Autodesk Inventor part; units mm, degrees
ref_plane "acrylic_sheet_plane" through (0, 0, 4) normal (0, 0, 1) x (1, 0, 0)
ref_plane "YZ Plane" through (0, 0, 0) normal (1, 0, 0) x (0, 1, 0)
ref_plane "XZ Plane" through (0, 0, 0) normal (0, 1, 0) x (-1, 0, 0)
sketch "ferrite_layer_outline_sketch" plane through (0, 0, 0) normal (0, 0, 1) x (1, 0, 0)
  line L0 (-400, 200) -> (400, 200)
  line L1 (400, 200) -> (400, -200)
  line L2 (400, -200) -> (-400, -200)
  line L3 (-400, -200) -> (-400, 200)
  line L4 (0, 200) -> (0, -200) construction
  line L5 (0, 136.1953) -> (0, -273.5408) construction
  line L6 (0, 200) -> (0, -200)
  point P0 (0, 0)
  point P1 (0, 0)
  point P2 (0, 0)
  dimension "d85" = 800
  dimension "d86" = 400
extrude "Sheet Extrude" add sketch "ferrite_layer_outline_sketch" along normal blind 4
ref_plane "acrylic_sheet_plane" through (0, 0, 4) normal (0, 0, 1) x (1, 0, 0)
sketch "Sketch4" plane through (0, 0, 4) normal (0, 0, 1) x (1, 0, 0)
  line L0 (-385.5, 109) -> (-370.5, 109)
  line L1 (-370.5, 109) -> (-370.5, -109)
  line L2 (-370.5, -109) -> (-385.5, -109)
  line L3 (-385.5, -109) -> (-385.5, 109)
  line L4 (-12.6534, 0) -> (47.471, 0)
  line L5 (-400, 200) -> (-400, -200)
  line L6 (400, 200) -> (-400, 200)
  line L7 (-400, -200) -> (400, -200)
  point P0 (0, 0)
  point P1 (-385.5, 0)
  point P2 (-400, 0)
  dimension "d43" = 15
  dimension "d44" = 218
  dimension "d45" = 14.5
extrude "Extrusion9" cut sketch "Sketch4" against normal through all
pattern_linear "Rectangular Pattern 7 fer" count 7 spacing 126 along (1, 0, 0) of "Extrusion9"
pattern_linear "Rectangular Pattern 8 fer" count 8 spacing 108 along (1, 0, 0) of "Extrusion9"
pattern_linear "pattern_test_#_of_ferrites 9 fer" [suppressed]
pattern_linear "Rectangular Pattern 10 fer" [suppressed]
pattern_linear "Rectangular Pattern 13" count 13 spacing 63 along (1, 0, 0) of "Extrusion9"
sketch "dimension_layout_sketch" plane through (0, 0, 4) normal (0, 0, 1) x (1, 0, 0)
  line L0 (-400, 200) -> (-400, -200)
  line L1 (400, -200) -> (400, 200)
  line L2 (400, 200) -> (-400, 200)
  line L3 (-400, -200) -> (400, -200)
  line L4 (-400, 150) -> (400, 150)
  line L5 (400, 150) -> (400, -150)
  line L6 (400, -150) -> (-400, -150)
  line L7 (-400, -150) -> (-400, 150)
  line L8 (0, 150) -> (0, -150) construction
  line L9 (-400, 200) -> (-400, -200) construction
  circle A0 centre (-359.2579, 182.7315) radius 4
  point P0 (0, 0)
  dimension "d87" = 300
  dimension "d88" = 8
sketch "wire_guide_layout_sketch" plane through (0, 0, 4) normal (0, 0, 1) x (1, 0, 0)
  line L0 (-400, -200) -> (400, -200)
  line L1 (-356.5, 92.3814) -> (-350, 92.3814)
  line L2 (-350, 92.3814) -> (-350, -200)
  line L3 (-350, -200) -> (-356.5, -200)
  line L4 (-356.5, -200) -> (-356.5, 92.3814)
  line L5 (-400, 200) -> (-400, -200)
  line L6 (-385.5, 109) -> (-370.5, 109)
  line L7 (-350, -60) -> (-345.5, -60)
  line L8 (-345.5, -60) -> (-345.5, -200)
  line L9 (-345.5, -200) -> (-350, -200)
  point P0 (0, 0)
  dimension "d89" = 43.5
  dimension "d90" = 6.5
  dimension "d91" = 140
  dimension "d92" = 4.5
extrude "wire_guide Cut" cut sketch "wire_guide_layout_sketch" against normal through all
equation "\"d85\" = track_length"
equation "\"d86\" = layer_width"
equation "\"d43\" = ferrite_width"
equation "\"d44\" = ferrite_length"
equation "\"d45\" = edge_gap_distance"
equation "\"d50\" = parameter_5"
equation "\"d62\" = test_parameter_5"
equation "\"d87\" = track_width"
equation "\"d88\" = bolt_diameter"
equation "\"track_length\" = 800"
equation "\"track_width\" = 300"
equation "\"edge_gap_distance\" = 14.5"
equation "\"ferrite_length\" = 218"
equation "\"ferrite_width\" = 15"
equation "\"number_of_ferrites\" = 7"
equation "\"acrylic_sheet_8mm\" = 8"
equation "\"layer_width\" = 400"
equation "\"bolt_diameter\" = 8"
equation "\"layer_length\" = 800"
equation "\"real_sheet_width\" = 500"
equation "\"ferrite_height\" = 8"
equation "\"parameter_2\" = 30"
equation "\"parameter_6\" = 120"
equation "\"number_of_bolts\" = 5"
equation "\"x_offset_for_bolts\" = 75"
equation "\"y_offset_for_bolts\" = 175"
equation "\"wire_diameter\" = 4.5"
equation "\"distance_between_wires\" = -1.2 * wire_diameter + 0.2 * parameter_6"
equation "\"distance_between_wires_edge\" = -1.5 * wire_diameter + 0.5 * parameter_2"
equation "\"bend_radius_inner\" = 15"
equation "\"wall_length\" = track_length"
equation "\"wall_width\" = -0.5 * track_width + 0.5 * layer_width"
equation "\"wall_thickness\" = 25"
properties part number "ferrite_layer_dex_1R1"
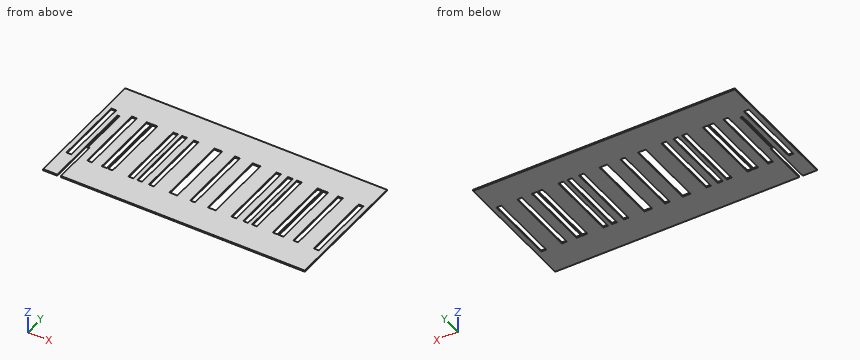
Could you check a few things on this model? Use its own coordinates, in mm. Give positions to 0.01 mm unless a question says otherwise; leave off trailing zeros. Order: outer loops, then holes, each group sorted by start corner. A loop starts at its lowest first (then second) coordinate and runs counter-clockwise, first axis right, second up.
Q1. Suppose I cut it at A-A, the plane x = -126. Write out the boundary of the cut face in (y, z).
Q2. Suppose I cut it at B-B, the plane y = 34. Count the separate pieces of the cut face and the enclosed holes in it, and give its area (3 significant figures).
Q3. If I drill on line 1 along Y through (x, z) = (-65, 1.9); line 2 along X through (y, z) = (-127.5, 3.55), over which ranges is the centre line in solid material (lowest first)?
Solution:
1. outline: (-200, 0) - (-109, 0) - (-109, 4) - (-200, 4) - close; (109, 0) - (200, 0) - (200, 4) - (109, 4) - close
2. separate pieces: 19
2. enclosed holes: 0
2. area: 2,080 mm2
3. line 1: y = -200 to -109, 109 to 200
3. line 2: x = -400 to -356.5, -345.5 to 400
